Source: CAD feature listing. Evaluate the final solid. Frame: model axes, mm. A direction names the side the tool comes from. Give positions to 0.01 mm unless a question says otherwise; leave off trailing zeros. Order: outer loops, then holes, each group sorted by start corner. A loop starts at its lowest first (then second) coordinate and runs counter-clockwise, first axis right, second up. Notation, with made-up numbers: (30.5, 33.5) -> (78.5, 33.5) arc R15 ccw to (78.5, 59.5) -> close; hole circle Ø7 at (44.25, 43.5). An arc over 180 degrees is marked (long way). Answer in a Markdown table with one row per item.
```python
from build123d import *

# Parameters (mm, degrees)
F0_R     = 18.65
F0_R_2   = 11.7
F1_DEPTH = 1.65
F3_DEPTH = 1.59
F5_DEPTH = 0.75
F6_R     = 0.5
F7_DEPTH = 10


with BuildPart() as f1:
    # F0 (on Top) → F1 (new body)
    with BuildSketch(Plane.XY):
        Circle(F0_R)
        Circle(F0_R_2, mode=Mode.SUBTRACT)
    extrude(amount=F1_DEPTH)

    # F2 (on face) → F3 (join)
    with BuildSketch(Plane.XY.offset(1.65)):
        Polygon((6.8182058502, 15.9798175517), (4.4516875758, 16.6139242122), (2.0851693014, 17.2480308727), (0.8169559804, 12.5149943239), (3.1834742548, 11.8808876634), (5.5499925292, 11.2467810029), align=None)
        Polygon((-6.8182058502, 15.9798175517), (-5.5499925292, 11.2467810029), (-3.1834742548, 11.8808876634), (-0.8169559804, 12.5149943239), (-2.0851693014, 17.2480308727), (-4.4516875758, 16.6139242122), align=None)
        Polygon((-13.8946482503, 10.4298250225), (-10.4298250225, 6.9650017947), (-8.6974134086, 8.6974134086), (-6.9650017947, 10.4298250225), (-10.4298250225, 13.8946482503), (-12.1622366364, 12.1622366364), align=None)
        Polygon((-17.2480308727, 2.0851693014), (-12.5149943239, 0.8169559804), (-11.8808876634, 3.1834742548), (-11.2467810029, 5.5499925292), (-15.9798175517, 6.8182058502), (-16.6139242122, 4.4516875758), align=None)
        Polygon((-15.9798175517, -6.8182058502), (-11.2467810029, -5.5499925292), (-11.8808876634, -3.1834742548), (-12.5149943239, -0.8169559804), (-17.2480308727, -2.0851693014), (-16.6139242122, -4.4516875758), align=None)
        Polygon((-10.4298250225, -13.8946482503), (-6.9650017947, -10.4298250225), (-8.6974134086, -8.6974134086), (-10.4298250225, -6.9650017947), (-13.8946482503, -10.4298250225), (-12.1622366364, -12.1622366364), align=None)
        Polygon((-2.0851693014, -17.2480308727), (-0.8169559804, -12.5149943239), (-3.1834742548, -11.8808876634), (-5.5499925292, -11.2467810029), (-6.8182058502, -15.9798175517), (-4.4516875758, -16.6139242122), align=None)
        Polygon((6.8182058502, -15.9798175517), (5.5499925292, -11.2467810029), (3.1834742548, -11.8808876634), (0.8169559804, -12.5149943239), (2.0851693014, -17.2480308727), (4.4516875758, -16.6139242122), align=None)
        Polygon((13.8946482503, -10.4298250225), (10.4298250225, -6.9650017947), (8.6974134086, -8.6974134086), (6.9650017947, -10.4298250225), (10.4298250225, -13.8946482503), (12.1622366364, -12.1622366364), align=None)
        Polygon((17.2480308727, -2.0851693014), (12.5149943239, -0.8169559804), (11.8808876634, -3.1834742548), (11.2467810029, -5.5499925292), (15.9798175517, -6.8182058502), (16.6139242122, -4.4516875758), align=None)
        Polygon((15.9798175517, 6.8182058502), (11.2467810029, 5.5499925292), (11.8808876634, 3.1834742548), (12.5149943239, 0.8169559804), (17.2480308727, 2.0851693014), (16.6139242122, 4.4516875758), align=None)
        Polygon((10.4298250225, 13.8946482503), (6.9650017947, 10.4298250225), (8.6974134086, 8.6974134086), (10.4298250225, 6.9650017947), (13.8946482503, 10.4298250225), (12.1622366364, 12.1622366364), align=None)
    extrude(amount=F3_DEPTH)

    # F4 (on face) → F5 (join)
    with BuildSketch(Plane.XY.offset(1.65)):
        Polygon((0.445, 17.38), (0, 17.38), (-0.445, 17.38), (-0.445, 15.73), (0, 15.73), (0.445, 15.73), align=None)
        Polygon((9.0753813047, 14.8290215178), (8.69, 15.0515215178), (8.3046186953, 15.2740215178), (7.4796186953, 13.8450796015), (7.865, 13.6225796015), (8.2503813047, 13.4000796015), align=None)
        Polygon((17.38, 0), (17.38, 0.445), (15.73, 0.445), (15.73, 0), (15.73, -0.445), (17.38, -0.445), align=None)
        Polygon((-15.73, 0.445), (-17.38, 0.445), (-17.38, 0), (-17.38, -0.445), (-15.73, -0.445), (-15.73, 0), align=None)
        Polygon((-7.4796186953, 13.8450796015), (-8.3046186953, 15.2740215178), (-8.69, 15.0515215178), (-9.0753813047, 14.8290215178), (-8.2503813047, 13.4000796015), (-7.865, 13.6225796015), align=None)
        Polygon((-8.2503813047, -13.4000796015), (-9.0753813047, -14.8290215178), (-8.69, -15.0515215178), (-8.3046186953, -15.2740215178), (-7.4796186953, -13.8450796015), (-7.865, -13.6225796015), align=None)
        Polygon((-0.445, -17.38), (0, -17.38), (0.445, -17.38), (0.445, -15.73), (0, -15.73), (-0.445, -15.73), align=None)
        Polygon((8.3046186953, -15.2740215178), (8.69, -15.0515215178), (9.0753813047, -14.8290215178), (8.2503813047, -13.4000796015), (7.865, -13.6225796015), (7.4796186953, -13.8450796015), align=None)
    extrude(amount=F5_DEPTH)

    # F6 (on face) → F7 (join)
    with BuildSketch(Plane(origin=(0, 0, 0), x_dir=(1, 0, 0), z_dir=(0, 0, -1))):
        with Locations((-15.0515215178, 8.69)):
            Circle(F6_R)
        with Locations((-15.0515215178, -8.69)):
            Circle(F6_R)
        with Locations((15.0515215178, -8.69)):
            Circle(F6_R)
        with Locations((15.0515215178, 8.69)):
            Circle(F6_R)
    extrude(amount=F7_DEPTH)


solid = f1.part
```
(1) Pull-direction query (X, two-part tool) for faces 4 (the flat face through (-13.646, -6.193, 2.434)), 5 (the flat face through (-14.848, -1.442, 2.434)), 6 (the flat face through (-6.175, -13.58, 2.434)), 7 (the flat face through (17, 0, 2.4)); classes: +X half, -X half, draft (parallel to the pull), parting line (faces both ways), or undercut.
A:
| item | result |
|---|---|
| face 4 | undercut |
| face 5 | -X half |
| face 6 | undercut |
| face 7 | draft |
(2) First-contact query: pin 1 Ø1.8 at (x, y) = (-8, -14.5) entering from +Z; pin 2 Ø2 at (x, z) = (12.5, -2.5) entering from +Y (3 decimals); pin 3 Ø3 at (y, z) = (-11.5, 1) entering from -X; pin 4 Ø0.6 at (x, z) = (0, 2) entering from +Y. Flat tips, straight axial feed; report the tip coordinate or a pass-through.
A:
| item | result |
|---|---|
| pin 1 | stops at z = 2.4 |
| pin 2 | passes through |
| pin 3 | stops at x = -15.74 |
| pin 4 | stops at y = 17.38 |
(3) Access query for faces 1 (the flat face through (-12.138, -8.673, 2.434)), 2 (the flat face through (6.175, 13.58, 2.434)), 3 (the flat face through (14.848, 1.442, 2.434)). Directions: +Z, -Z, +X, -X, +Y, -Y. A direction counts if a zero-diameter tool reaches every point of the face in a straight line with its end or side. Return the directions, or none.
A:
| item | result |
|---|---|
| face 1 | +Z, -X |
| face 2 | +Z |
| face 3 | +Z, +X |
(4) Section query A-A (x = 0). Return the cut outline in (y, z).
A:
| item | result |
|---|---|
| outline | (-18.65, 0) -> (-11.7, 0) -> (-11.7, 1.65) -> (-15.73, 1.65) -> (-15.73, 2.4) -> (-17.38, 2.4) -> (-17.38, 1.65) -> (-18.65, 1.65) -> close; (11.7, 0) -> (18.65, 0) -> (18.65, 1.65) -> (17.38, 1.65) -> (17.38, 2.4) -> (15.73, 2.4) -> (15.73, 1.65) -> (11.7, 1.65) -> close |
(5) Section query D-D (z = 1). Return the cut outline in (x, y).
A:
| item | result |
|---|---|
| outline | circle Ø37.3 at (0, 0); hole circle Ø23.4 at (0, 0) |
(6) Section query C-C (z = -9). Return the cut outline in (x, y).
A:
| item | result |
|---|---|
| outline | circle Ø1 at (-15.05, -8.69); circle Ø1 at (-15.05, 8.69); circle Ø1 at (15.05, -8.69); circle Ø1 at (15.05, 8.69) |
(7) Ray query, probe 1 along Y at (x, z) = (0, 1.3); probe 2 along Z at (x, y) = (-16.5, -1.5); probe 3 along Z at (x, y) = (-11, 8). Return the intervals inside material, ascending.
A:
| item | result |
|---|---|
| probe 1 | y = -18.65 to -11.7, 11.7 to 18.65 |
| probe 2 | z = 0 to 1.65 |
| probe 3 | z = 0 to 3.24 |
